```python
from build123d import *

# Parameters (mm, degrees)
F0_R     = 6.35
F1_DEPTH = 38.1


with BuildPart() as f1:
    # F0 (on Right) → F1 (new body)
    with BuildSketch(Plane.YZ):
        with BuildLine():
            Line((-5.499261, 3.888647), (5.499261, 3.888647))
            Line((5.499261, 3.888647), (10.411803, 12.397418))
            ThreePointArc((10.411803, 12.397418), (9.825083, 13.413647), (10.411803, 14.429875))
            Line((10.411803, 14.429875), (5.499261, 22.938647))
            Line((5.499261, 22.938647), (-5.499261, 22.938647))
            Line((-5.499261, 22.938647), (-10.998523, 13.413647))
            Line((-10.998523, 13.413647), (-5.499261, 3.888647))
        make_face()
        with Locations((0, 13.413647)):
            Circle(F0_R, mode=Mode.SUBTRACT)
    extrude(amount=F1_DEPTH)


solid = f1.part
```
CAD build for the part. Positions are in the model's coordinates, mm. Round coordinates to 2 decimals unless told otherwise and drop trailing zeros. Loops run counter-clockwise (first coordinate to the right, second up) from the corner with the lowest first, then second, coordinate; pieces in that order, holes last. Notation, with made-up numbers: M 52,79.25 L 87,79.25 A23 ccw 87,118.25 Z; hole C 18,83.25 d1. An arc over 180 degrees is marked long. Use a Markdown table: item, result. Add a question column.
(1) Cut at A-A (y = 0). Give the cut face in (x, z).
(2) Flat gauge pins, fed straight in: pin 1 (2 mm diameter, centred on x = 21.5, z = 19.5, fed in from +Y); pin 2 (1.5 mm diameter, centred on x = 27.5, z = 6.5, fed in from +Y); pin 3 (6 mm diameter, centred on x = 31, z = 13, fed in from +Y). Where does each tip first touch, or does it go through?
(3) Cut at D-D (z = 20.25). Give the cut face in (x, y).
(4) Cut at C-C (z = 9). Give the cut face in (x, y).
(5) Cut at B-B (x = 2). Give the cut face in (y, z), and give its area (3 significant figures).
(6) Drill centre lines: line 1 (Z direction, x = 11, y = 0); line 2 (Z direction, x = 17, y = -1.25); line 3 (Y direction, x = 7.5, z = 15.5). Where is each one in solid material? Low to high.
(7) Pull direction Y, two halves, no side cores. Call faces 1 (the face through (18.78, -8.21, 18.24)), 2 (the face through (38.1, 0, 20)), 3 (the face through (18.783, 7.99, 18.625)), 4 (the face through (18.783, -1.377, 7.215)): +Y half, -Y half, draft (parallel to the pull), parting line (faces both ways), or undercut.
Geometry says:
| question | item | result |
|---|---|---|
| 1 | outline | M 0,3.89 L 38.1,3.89 L 38.1,7.06 L 0,7.06 Z; M 0,19.76 L 38.1,19.76 L 38.1,22.94 L 0,22.94 Z |
| 2 | pin 1 | stops at y = 8.06 |
| 2 | pin 2 | stops at y = 7.44 |
| 2 | pin 3 | stops at y = 10.41 |
| 3 | outline | M 0,-7.05 L 38.1,-7.05 L 38.1,7.05 L 0,7.05 Z |
| 4 | outline | M 0,-8.45 L 38.1,-8.45 L 38.1,-4.57 L 0,-4.57 Z; M 0,4.57 L 38.1,4.57 L 38.1,8.45 L 0,8.45 Z |
| 5 | outline | M -11,13.41 L -5.5,3.89 L 5.5,3.89 L 10.41,12.4 A1.17 cw 10.41,14.43 L 5.5,22.94 L -5.5,22.94 Z; hole C 0,13.41 d12.7 |
| 5 | area | 186 mm² |
| 6 | line 1 | z = 3.89 to 7.06, 19.76 to 22.94 |
| 6 | line 2 | z = 3.89 to 7.19, 19.64 to 22.94 |
| 6 | line 3 | y = -9.79 to -6, 6 to 9.79 |
| 7 | face 1 | -Y half |
| 7 | face 2 | draft |
| 7 | face 3 | +Y half |
| 7 | face 4 | undercut |
